Answer from the drawing. Dimensions are ordinates in mm from the lowest x, y and z of the part. Give positions to 0.01 mm unless a question says otherwise; leave off trailing zeros. Loops run counter-clockwise (first coordinate to the right, second up) from the corner with the lowest first, then second, coordinate; pieces in that order, holes last.
Item 1: Consider line 1 along X through (y, z) = (18, 57.5); line 2 along X through (y, z) = (10, 175.5). Determine where each line is inside the solid, lowest interval first.
Item 2: The mould has two halves that part along Y. Classify the marked faces 1, 2 and 3: pulls with the +Y half, pulls with the -Y half, needs draft (parallel to the pull), parting line crosses it, or undercut.
Item 3: Section A-A, the plane z = 19 is taken. Give the vertices of the cut face in (x, y).
Item 4: Each of these flat-tipped pins is pushed along its axis until it touches: pin 1 Ø4 at (y, z) = (13.5, 26.5) entering from +X; pin 2 Ø13.5 at (x, z) = (26, 46.5) entering from +Y; pin 3 Ø2 at (x, z) = (10.5, 76.5) entering from +Y. Where does it stop, or does it pass through?
Item 5: Section B-B, the plane x = 34.5 is taken. Give the vertices of the cut face in (y, z), and give its area (3 significant figures).
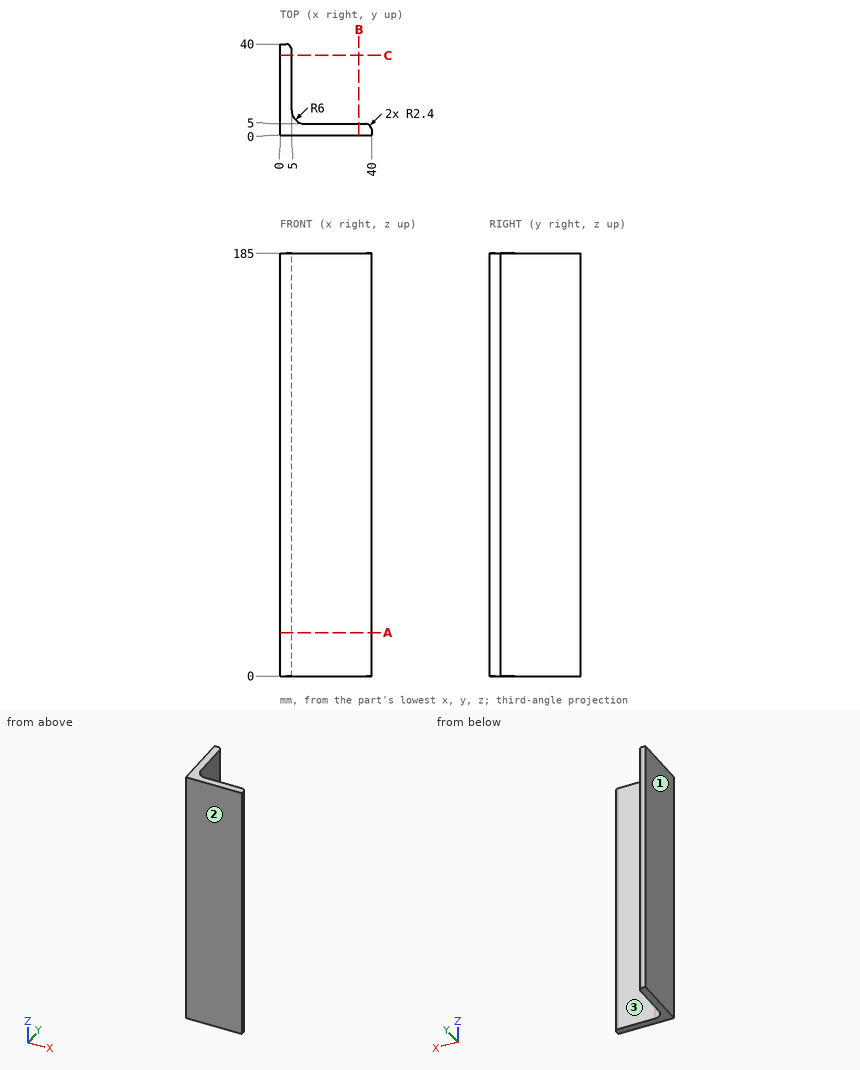
Worked answers:
1. line 1: x = 0 to 5
1. line 2: x = 0 to 5.08
2. face 1: needs draft
2. face 2: pulls with the -Y half
2. face 3: pulls with the +Y half
3. outline: (0, 0) - (40, 0) - (40, 2.6) arc R2.4 ccw to (37.6, 5) - (11, 5) arc R6 cw to (5, 11) - (5, 37.6) arc R2.4 ccw to (2.6, 40) - (0, 40) - close
4. pin 1: stops at x = 5
4. pin 2: stops at y = 5
4. pin 3: stops at y = 5.19
5. outline: (0, 0) - (5, 0) - (5, 185) - (0, 185) - close
5. area: 925 mm2
